Part model, mm, in its own coordinate system. Give positions to 0.01 mm unless a question says otherwise; leave off trailing zeros. Order: outer loops, then holes, each group sorted by start corner. A loop starts at its lowest first (then second) coordinate and runs counter-clockwise, first axis right, second up. Notation, with made-up numbers: (-1.75, -38) - (48.25, -38) arc R18 cw to (48.25, -30) - close; hole circle Ø11 at (4, -36). An arc over 180 degrees is marked (long way). One line per item, written item: value.
```python
from build123d import *

# Parameters (mm, degrees)
F0_R     = 4.75
F0_R_2   = 1.5
F1_DEPTH = 5


with BuildPart() as f1:
    # F0 (on Top) → F1 (new body)
    with BuildSketch(Plane.XY):
        with BuildLine():
            ThreePointArc((8, 0), (6.483766, 4.686233), (2.509804, 7.59611))
            ThreePointArc((2.509804, 7.59611), (-8, 0), (2.509804, -7.59611))
            ThreePointArc((2.509804, -7.59611), (6.483766, -4.686233), (8, 0))
        make_face()
        Circle(F0_R, mode=Mode.SUBTRACT)
        with BuildLine():
            ThreePointArc((14.004902, -3.798055), (16.75, 0), (14.004902, 3.798055))
            Line((14.004902, 3.798055), (2.509804, 7.59611))
            ThreePointArc((2.509804, 7.59611), (6.483766, 4.686233), (8, 0))
            ThreePointArc((8, 0), (6.483766, -4.686233), (2.509804, -7.59611))
            Line((2.509804, -7.59611), (14.004902, -3.798055))
        make_face()
        with Locations((12.75, 0)):
            Circle(F0_R_2, mode=Mode.SUBTRACT)
    extrude(amount=F1_DEPTH)


solid = f1.part
```
1) Drop flat-ended pins along their axis: P1, Ø2, axis at y = 6, z = 2.5, coming from the -X side (3 decimals); P2, Ø1, axis at x = 8, y = 0.5, coming from the -Z side; P3, Ø1.5, axis at x = 4, z = 0.5, coming from the -Y side. Give the stop position or say it passes through.
Answer:
P1: stops at x = -6.245
P2: stops at z = 0
P3: stops at y = -7.35
2) Wall check: line 1 along Y through (x, z) = (0, 3.5); line 2 along Y through (x, z) = (12.75, 3.9); line 3 along X through (y, z) = (0.75, 1.25). Give the ranges that are in metal, low to high. Write a range as [from, to].
Answer:
line 1: y = [-8, -4.75], [4.75, 8]
line 2: y = [-4.21, -1.5], [1.5, 4.21]
line 3: x = [-7.96, -4.69], [4.69, 11.45], [14.05, 16.68]
3) Two-plate mould, pull along X, no slides. Class faces 1 (the face through (7, 0, 5)), 2 (the face through (-8, 0, 2)), 3 (the face through (2.192, -4.214, 2.465)): pulls with the +X half, pulls with the -X half, needs draft (parallel to the pull), parting line crosses it, or undercut.
Answer:
face 1: needs draft
face 2: parting line crosses it
face 3: undercut
4) Slice it at A-A on x = 0. Write the cut outline in (y, z).
Answer:
outline: (-8, 0) - (-4.75, 0) - (-4.75, 5) - (-8, 5) - close; (4.75, 0) - (8, 0) - (8, 5) - (4.75, 5) - close
5) Slice it at C-C on y = 0. Write the cut outline in (x, z), then the cut area to 4 significant figures.
Answer:
outline: (-8, 0) - (-4.75, 0) - (-4.75, 5) - (-8, 5) - close; (4.75, 0) - (11.25, 0) - (11.25, 5) - (4.75, 5) - close; (14.25, 0) - (16.75, 0) - (16.75, 5) - (14.25, 5) - close
area: 61.25 mm2
6) Slice it at B-B on y = -2.75. Write the cut outline in (x, z).
Answer:
outline: (-7.51, 0) - (-3.87, 0) - (-3.87, 5) - (-7.51, 5) - close; (3.87, 0) - (15.65, 0) - (15.65, 5) - (3.87, 5) - close
7) Slice it at D-D on z = 2.65. Write the cut outline in (x, y), then the cut area to 3 significant figures.
Answer:
outline: (2.51, -7.6) - (14, -3.8) arc R4 ccw to (14, 3.8) - (2.51, 7.6) arc R8 ccw (long way) to start; hole circle Ø9.5 at (0, 0); hole circle Ø3 at (12.75, 0)
area: 208 mm2
